Source: CAD feature listing. Evaluate the final solid. Frame: model axes, mm. A direction names the side the tool comes from. Coordinates: 2 decimals unless noted, no trailing zeros. Loops run counter-clockwise (first coordinate to the right, second up) from the corner with the lowest first, then second, coordinate; pieces in that order, holes last. Notation, with made-up numbers: M 3,6.5 L 50,6.5 A17 ccw 50,28.5 Z; hole C 50.5,-32.75 d11. An arc over 180 degrees is marked long. One line per question, with ' | ' between items. Start each with the question number.
1. Section query A-A, the plane x = -13.5. Output: boundary loops of the cut face in (y, z), and give its area (3 significant figures).
2. Section query C-C, the plane y = 0. Output: boundary loops of the cut face in (x, z).
3. Ray query, probe 1 along Y at (x, z) = (13.5, 0.7); probe 2 along Y at (x, z) = (-14.5, 1); probe 3 along Z at (x, y) = (-4.5, -6). Return the intervals inside material, ascending.
4. Access query for faces 5 (the flat face through (0, -8, 0)), 6 (the cylindrical face through (-12.946, -14.565, 1.479)). Directions: +Z, -Z, +X, -X, +Y, -Y. A direction counts if a zero-diameter tool reaches every point of the face in a straight line with its end or side. Return the directions, or none.
5. Pin query (flat end, axial travel): P1, Ø3, axis at x = 13.5, y = -13.5, coming from the +Z side; P2, Ø8, axis at x = -3.5, z = -11, coming from the +Y side; P3, Ø4, axis at x = -9, y = -14.5, coming from the -Z side; P4, Ø1, axis at x = 14.5, z = -1, coming from the +Y side. Return the tip coordinate at first contact, or that it passes through.
6. Mould query, pull axis X, two halves, no side actions, for faces 1 (the cylindrical face through (-12.946, 12.435, 1.479)), 2 (the flat face through (19, 0, 1)), 3 (the flat face through (0, 19, 1)), 4 (the cylindrical face through (-6.466, -2.681, -7.395)). Classes: pulls with the +X half, pulls with the -X half, needs draft (parallel to the pull), parting line crosses it, or undercut.
```python
from build123d import *

# Parameters (mm, degrees)
SKETCH_1_W      = 38
SKETCH_1_H      = 38
SKETCH_1_R      = 1.2
EXTRUDE_1_DEPTH = 3
SKETCH_2_R      = 7
EXTRUDE_2_DEPTH = 15


with BuildPart() as part:
    # 草图1 → 凸台-拉伸1 (new body)
    with BuildSketch(Plane.XY):
        Rectangle(SKETCH_1_W, SKETCH_1_H)
        with Locations((-13.5, 13.5)):
            Circle(SKETCH_1_R, mode=Mode.SUBTRACT)
        with Locations((13.5, 13.5)):
            Circle(SKETCH_1_R, mode=Mode.SUBTRACT)
        with Locations((13.5, -13.5)):
            Circle(SKETCH_1_R, mode=Mode.SUBTRACT)
        with Locations((-13.5, -13.5)):
            Circle(SKETCH_1_R, mode=Mode.SUBTRACT)
    extrude(amount=EXTRUDE_1_DEPTH)

    # 草图2 → 凸台-拉伸2 (add)
    with BuildSketch(Plane(origin=(0, 0, 0), x_dir=(-1, 0, 0), z_dir=(0, 0, -1))):
        Circle(SKETCH_2_R)
    extrude(amount=EXTRUDE_2_DEPTH)


solid = part.part
```
Taken from the geometry:
1) outline: M -19,0 L -14.7,0 L -14.7,3 L -19,3 Z; M -12.3,0 L 12.3,0 L 12.3,3 L -12.3,3 Z; M 14.7,0 L 19,0 L 19,3 L 14.7,3 Z | area: 99.6 mm^2
2) outline: M -19,0 L -7,0 L -7,-15 L 7,-15 L 7,0 L 19,0 L 19,3 L -19,3 Z
3) probe 1: -19 to -14.7, -12.3 to 12.3, 14.7 to 19 | probe 2: -19 to -14.16, -12.84 to 12.84, 14.16 to 19 | probe 3: 0 to 3
4) face 5: -Z | face 6: +Z, -Z
5) P1: z = 3 | P2: y = 7 | P3: z = 0 | P4: through
6) face 1: undercut | face 2: pulls with the +X half | face 3: needs draft | face 4: parting line crosses it
